```python
from build123d import *

# Parameters (mm, degrees)
SKETCH1_W                = 44.48
SKETCH1_H                = 4.5
SKETCH1_R                = 1.5
BOSS_EXTRUDE1_DEPTH      = 3
BOSS_EXTRUDE2_DEPTH      = 15
BOSS_EXTRUDE2_DEPTH_BACK = 2
BOSS_EXTRUDE3_DEPTH      = 2.25
CUT_EXTRUDE1_DEPTH       = 44.517933829
CUT_EXTRUDE1_DEPTH_BACK  = 44.517933829
SKETCH3_R                = 1.258736144


with BuildPart() as part:
    # Sketch1 → Boss-Extrude1 (new body)
    with BuildSketch(Plane(origin=(0, 0, 0), x_dir=(1, 0, 0), z_dir=(0, 1, 0))):
        Rectangle(SKETCH1_W, SKETCH1_H)
        with Locations(Location((-18.24, 0, 0), (0, 0, 270))):
            Circle(SKETCH1_R, mode=Mode.SUBTRACT)
        with Locations(Location((18.24, 0, 0), (0, 0, 270))):
            Circle(SKETCH1_R, mode=Mode.SUBTRACT)
    extrude(amount=BOSS_EXTRUDE1_DEPTH)

    # Sketch2 → Boss-Extrude2 (add, two sides: drawn at the far end of the back side and taken through both)
    with BuildSketch(Plane.XY.offset(-BOSS_EXTRUDE2_DEPTH_BACK)):
        with BuildLine():
            Line((-2.5, 34.266499161), (-2.5, 29.266499161))
            ThreePointArc((-2.5, 29.266499161), (-1.752753406, 29.385733282), (-1, 29.462912018))
            Line((-1, 29.462912018), (-1, 34.266499161))
            Line((-1, 34.266499161), (-2.5, 34.266499161))
        make_face()
        with BuildLine():
            Line((1, 34.266499161), (1, 29.462912018))
            ThreePointArc((1, 29.462912018), (1.752753406, 29.385733282), (2.5, 29.266499161))
            Line((2.5, 29.266499161), (2.5, 34.266499161))
            Line((2.5, 34.266499161), (1, 34.266499161))
        make_face()
        with BuildLine():
            ThreePointArc((-2.5, 29.266499161), (-10.392304845, 24.61684397), (-13.5, 16))
            ThreePointArc((-13.5, 16), (-10.756178265, 7.841897946), (-3.640054945, 3))
            ThreePointArc((-3.640054945, 3), (0, 2.5), (3.640054945, 3))
            ThreePointArc((3.640054945, 3), (10.756178265, 7.841897946), (13.5, 16))
            ThreePointArc((13.5, 16), (10.392304845, 24.61684397), (2.5, 29.266499161))
            ThreePointArc((2.5, 29.266499161), (1.752753406, 29.385733282), (1, 29.462912018))
            Line((1, 29.462912018), (1, 28.058606885))
            ThreePointArc((1, 28.058606885), (8.902527731, 24.194815434), (12.1, 16))
            ThreePointArc((12.1, 16), (-8.194815434, 7.097472269), (-1, 28.058606885))
            Line((-1, 28.058606885), (-1, 29.462912018))
            ThreePointArc((-1, 29.462912018), (-1.752753406, 29.385733282), (-2.5, 29.266499161))
        make_face()
    extrude(amount=BOSS_EXTRUDE2_DEPTH + BOSS_EXTRUDE2_DEPTH_BACK)

    # Sketch2_3 → Boss-Extrude3 (add, symmetric)
    with BuildSketch(Plane.XY):
        with BuildLine():
            ThreePointArc((13.5, 16), (10.756178265, 7.841897946), (3.640054945, 3))
            Line((3.640054945, 3), (13.5, 3))
            Line((13.5, 3), (13.5, 16))
        make_face()
        with BuildLine():
            ThreePointArc((-3.640054945, 3), (-10.756178265, 7.841897946), (-13.5, 16))
            Line((-13.5, 16), (-13.5, 3))
            Line((-13.5, 3), (-3.640054945, 3))
        make_face()
    extrude(amount=BOSS_EXTRUDE3_DEPTH, both=True)

    # Sketch3 → Cut-Extrude1 (cut, two sides: drawn at the far end of the back side and taken through both)
    with BuildSketch(Plane(origin=(0, 0, 0), x_dir=(0, 0, -1), z_dir=(1, 0, 0)).offset(-CUT_EXTRUDE1_DEPTH_BACK)):
        with Locations(Location((-6.5, 31.766499161, 0), (0, 0, 270))):
            Circle(SKETCH3_R)
    extrude(amount=CUT_EXTRUDE1_DEPTH + CUT_EXTRUDE1_DEPTH_BACK, mode=Mode.SUBTRACT)


solid = part.part
```
Could you check a few things on this model? Use its own coordinates, in mm. A direction names the side the tool comes from. Give positions to 0.01 mm unless a question says otherwise; leave off trailing zeros. Loops run counter-clockwise (first coordinate to the right, second up) from the corner with the lowest first, then second, coordinate; pieces in that order, holes last. Notation, with made-up numbers: (57.25, 55.25) - (103.25, 55.25) arc R30 cw to (103.25, 94.25) - close; hole circle Ø7 at (-26, -31). An arc over 180 degrees is marked (long way). Use one line per item in the form item = value.
1. I want a section at C-C (z = 12.25). Please give me the cut outline in (x, y).
Response values:
outline = (-2.5, 29.27) arc R13.5 ccw (long way) to (2.5, 29.27) - (2.5, 34.27) - (1, 34.27) - (1, 28.06) arc R12.1 cw (long way) to (-1, 28.06) - (-1, 34.27) - (-2.5, 34.27) - close
2. Thinking about a two-plate mould opening in X: for faces 1 (the face through (-2.5, 30, 6)), 2 (the face through (-2, 34.266, 6)), 3 (the face through (-19.704, 1.479, -0.325)), 4 (the face through (1, 30, 6)), which applies, released by +X, released by -X, zero draft, split by the parting line, or undercut?
Response values:
face_1 = released by -X
face_2 = zero draft
face_3 = undercut
face_4 = undercut
3. I want a section at D-D (z = 0.5). Please give me the cut outline in (x, y), and give its area (3 significant figures).
Response values:
outline = (-22.24, 0) - (-19.65, 0) - (-19.65, 3) - (-22.24, 3) - close; (-16.83, 0) - (16.83, 0) - (16.83, 3) - (13.5, 3) - (13.5, 16) arc R13.5 ccw to (2.5, 29.27) - (2.5, 34.27) - (1, 34.27) - (1, 28.06) arc R12.1 cw (long way) to (-1, 28.06) - (-1, 34.27) - (-2.5, 34.27) - (-2.5, 29.27) arc R13.5 ccw to (-13.5, 16) - (-13.5, 3) - (-16.83, 3) - close; (19.65, 0) - (22.24, 0) - (22.24, 3) - (19.65, 3) - close
area = 306 mm²
4. On a 3-axis mill with a long thin cutter (end or side, diameter ignored), from which of +Z, -Z, +X, -X, +Y, -Y can I reach the whole of each face in a straight line? I mean faces 5 (the face through (-3, 28, -2)), 6 (the face through (2.5, 33.4, 6.4)), 7 (the face through (-1, 30, 6)). Say none if no direction works.
Response values:
face_5 = -Z, +Y
face_6 = +Z, -Z, +X, +Y
face_7 = +Z, -Z, +Y
5. I want a section at B-B (y = 17). Please give me the cut outline in (x, z), and give its area (3 significant figures).
Response values:
outline = (-13.46, -2) - (-12.06, -2) - (-12.06, 15) - (-13.46, 15) - close; (12.06, -2) - (13.46, -2) - (13.46, 15) - (12.06, 15) - close
area = 47.7 mm²
6. I need wall thicknesses on probe 1 along X at (y, z) = (1.8, 0); probe 2 along X at (y, z) = (29.5, -1.5); probe 3 along X at (y, z) = (16, 9.5). Which ranges of each line are inside material? Lowest first, please.
Response values:
probe_1 = -22.24 to -19.74, -16.74 to 16.74, 19.74 to 22.24
probe_2 = -2.5 to -1, 1 to 2.5
probe_3 = -13.5 to -12.1, 12.1 to 13.5
7. I'm going to push flat-ended pins straight in: pin 1 Ø10 at (y, z) = (19, 12.5) entering from -X; pin 2 Ø6 at (y, z) = (18, 7.5) entering from +X; pin 3 Ø3 at (x, z) = (-7.5, 9.5) entering from +Y. Where does each tip first touch, or does it pass through?
Response values:
pin_1 = -13.5
pin_2 = 13.5
pin_3 = 28.09
8. I want a section at A-A (x = -18.24). Please give me the cut outline in (y, z).
Response values:
outline = (0, -2.25) - (3, -2.25) - (3, -1.5) - (0, -1.5) - close; (0, 1.5) - (3, 1.5) - (3, 2.25) - (0, 2.25) - close
